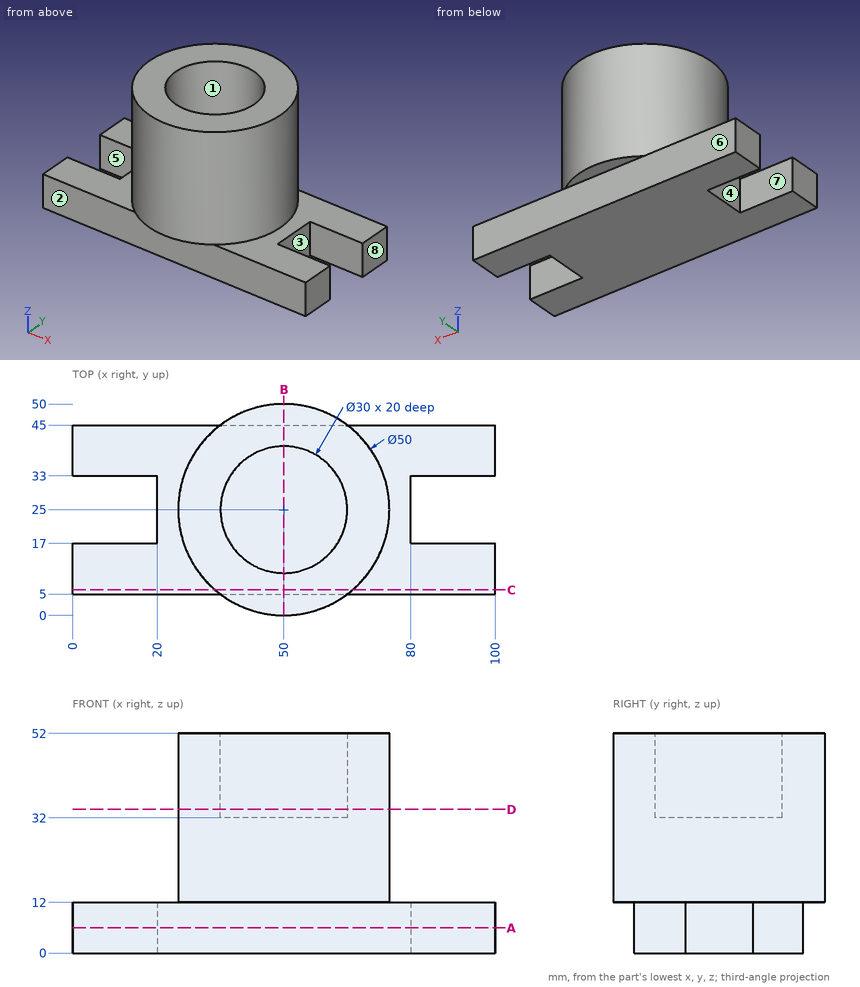
Verification items for this drawing (mm, ordinates from the low corner). A direction names the side the tool comes from. Coordinates: 2 decimals unless noted, no trailing zeros. Order: outer loops, then holes, each group sorted by start corner. A loop starts at its lowest first (then second) coordinate and runs counter-clockwise, first axis right, second up. Notation, with made-up numbers: (57.5, 60.5) -> (74.5, 60.5) arc R13 ccw to (74.5, 85.5) -> close; hole circle Ø10 at (87.25, -24). An arc over 180 degrees is marked (long way). Answer as CSV lines item,"result". Start each with the question number.
1) Material ranges on L1, parallel to Y at x = 87, z = 7; L2, parallel to Y at x = 50, z = 42; L3, parallel to Z at x = 75.5, y = 41, recorded low to high. Write a range as [from, to].
2) Cross-section at B-B, the plane x = 50. Record the boundary of the cut face in (y, z).
3) Release check for a two-part mould opening along Y. For the marked faces 5, 6, 7 and 8 record: released by +Y, released by -Y, zero draft, split by the parting line, or undercut.
4) Cross-section at A-A, the plane z = 6. Record the boundary of the cut face in (x, y), then the cut area to 3 significant figures.
5) Gauge pin test, flat ends, axial feed: pin 1 Ø1.5 at (x, y) = (51.5, 3) entering from -Z; pin 2 Ø1 at (x, z) = (28.5, 11.5) entering from -Y; pin 3 Ø6 at (y, z) = (25.5, 7.5) entering from -X; pin 4 Ø8 at (x, y) = (32, 23.5) entering from -Z. Record the tip position at first contact, or that the pin passes through.
6) Cross-section at C-C, the plane y = 6. Record the boundary of the cut face in (x, z), then the cut area to 3 significant figures.
7) Set-up check for the marked faces 1, 2, 3 and 4: record each of +Z, -Z, +X, -X, +Y, -Y from which the full face is reachable in a straight line by a thin tool's end or side.
8) Cross-section at D-D, the plane z = 34. Record the boundary of the cut face in (x, y), then the cut area to 3 significant figures.
Conclusion:
1,L1,"y = [5, 17], [33, 45]"
1,L2,"y = [0, 10], [40, 50]"
1,L3,"z = [0, 12]"
2,outline,"(0, 12) -> (5, 12) -> (5, 0) -> (45, 0) -> (45, 12) -> (50, 12) -> (50, 52) -> (40, 52) -> (40, 32) -> (10, 32) -> (10, 52) -> (0, 52) -> close"
3,face 5,"undercut"
3,face 6,"released by +Y"
3,face 7,"undercut"
3,face 8,"zero draft"
4,outline,"(0, 5) -> (100, 5) -> (100, 17) -> (80, 17) -> (80, 33) -> (100, 33) -> (100, 45) -> (0, 45) -> (0, 33) -> (20, 33) -> (20, 17) -> (0, 17) -> close"
4,area,"3,360 mm²"
5,pin 1,"stops at z = 12"
5,pin 2,"stops at y = 5"
5,pin 3,"stops at x = 20"
5,pin 4,"stops at z = 0"
6,outline,"(0, 0) -> (100, 0) -> (100, 12) -> (66.25, 12) -> (66.25, 52) -> (33.75, 52) -> (33.75, 12) -> (0, 12) -> close"
6,area,"2,500 mm²"
7,face 1,"+Z"
7,face 2,"-Z, +X, -X, -Y"
7,face 3,"+Z, -Z, +X"
7,face 4,"+Z, -Z, -X"
8,outline,"circle Ø50 at (50, 25); hole circle Ø30 at (50, 25)"
8,area,"1,260 mm²"
